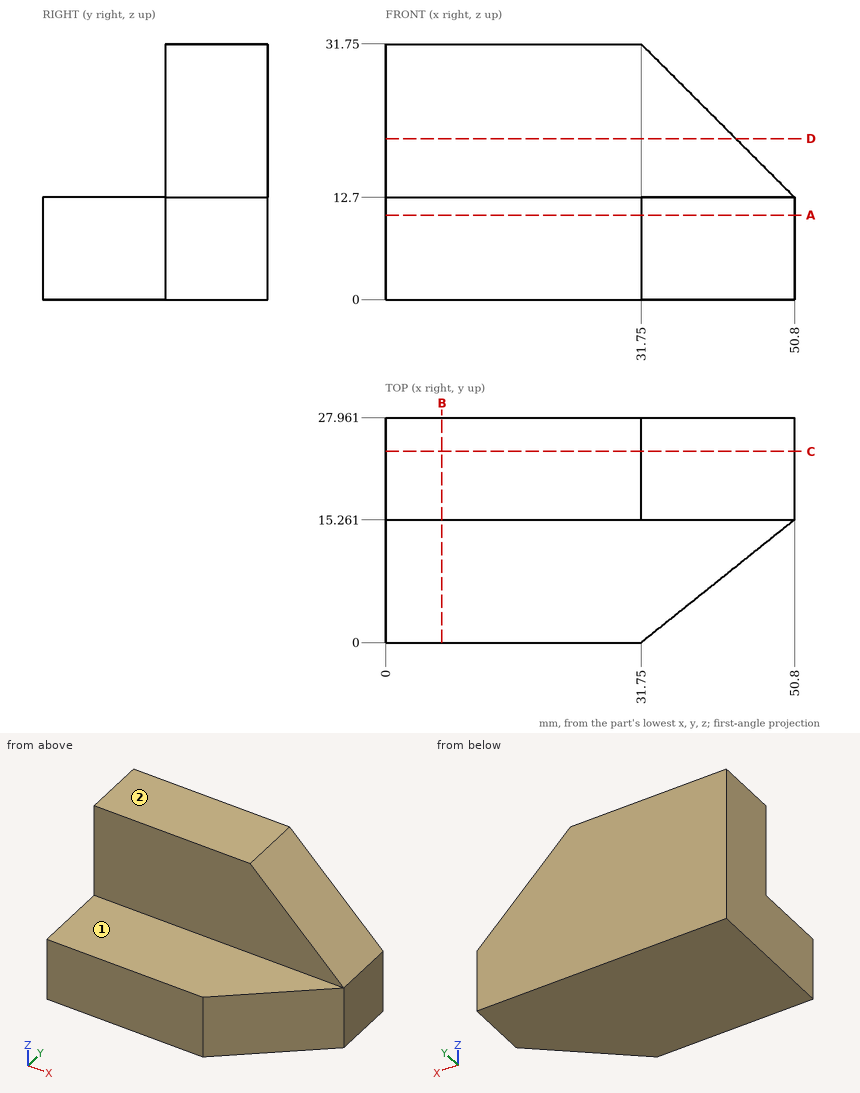
Print and shaded views of the part. All mm, measured from the part's lowest x, y and z. A direction names the side the tool comes from. Give positions to 0.01 mm unless a question says otherwise; leave off trailing zeros. Loops run counter-clockwise (first coordinate to the right, second up) from the corner with the lowest first, then second, coordinate; pieces in that order, holes last.
1) Flat gauge pins, fed straight in: pin 1 Ø12 at (x, y) = (26, 4) entering from +Z; pin 2 Ø8 at (x, y) = (38, 20) entering from +Z; pin 3 Ø12 at (x, z) = (41, 28.5) entering from -Y; pin 4 Ø10 at (y, z) = (8.5, 25.5) entering from +X (3 decimals). Where does each tip first touch, or does it go through?
2) Saw through at D-D (z = 20). Write the cut outline in (x, y).
3) Saw through at C-C (y = 23.75). Write the cut outline in (x, z).
4) Saw through at A-A (z = 10.5). Write the cut outline in (x, y).
5) Saw through at B-B (x = 7). Write the cut outline in (y, z).
6) Wall check: line 1 (Z direction, x = 11, y = 14.25); line 2 (Y direction, x = 43, z = 13); line 3 (Y direction, x = 40, z = 8). Give the ranges that are in metal, low to high.
7) Tool access for the marked faces 1 and 2: list every direction of +Z, -Z, +X, -X, +Y, -Y with a clear straight run to the whole face (end or side of a thin tool).
Answer block:
1. pin 1: stops at z = 12.7
1. pin 2: stops at z = 29.5
1. pin 3: stops at y = 15.26
1. pin 4: passes through
2. outline: (0, 15.26) - (43.5, 15.26) - (43.5, 27.96) - (0, 27.96) - close
3. outline: (0, 0) - (50.8, 0) - (50.8, 12.7) - (31.75, 31.75) - (0, 31.75) - close
4. outline: (0, 0) - (31.75, 0) - (50.8, 15.26) - (50.8, 27.96) - (0, 27.96) - close
5. outline: (0, 0) - (27.96, 0) - (27.96, 31.75) - (15.26, 31.75) - (15.26, 12.7) - (0, 12.7) - close
6. line 1: z = 0 to 12.7
6. line 2: y = 15.26 to 27.96
6. line 3: y = 6.61 to 27.96
7. face 1: +Z, +X, -X, -Y
7. face 2: +Z, +X, -X, +Y, -Y
